from build123d import *

# Parameters (mm, degrees)
EXTRUDE_1_DEPTH = 5


with BuildPart() as part:
    # 草图1 → 凸台-拉伸1 (new body)
    with BuildSketch(Plane(origin=(0, 0, 0), x_dir=(1, 0, 0), z_dir=(0, 1, 0))):
        with BuildLine():
            ThreePointArc((-46.803501746, 8.133377636), (-74.235016913, -2.264931442), (-44.950167705, -4))
            Line((-44.950167705, -4), (-59.407, -4))
            ThreePointArc((-59.407, -4), (-63.361137843, -0.603981718), (-60.601113484, 3.817603042))
            Line((-60.601113484, 3.817603042), (-46.803501746, 8.133377636))
        make_face()
        with BuildLine():
            Line((-60.13775005, 13.480207875), (-65.265019195, 2.816666667))
            ThreePointArc((-65.265019195, 2.816666667), (-65.892913632, 0.427696579), (-65.584160854, -2.023038254))
            Line((-65.584160854, -2.023038254), (-72.827832577, 1.459881143))
            ThreePointArc((-72.827832577, 1.459881143), (-68.690796982, 9.801077165), (-60.13775005, 13.480207875))
        make_face(mode=Mode.SUBTRACT)
        with BuildLine():
            Line((-72.887207875, -0.73075005), (-62.223666667, -5.858019195))
            ThreePointArc((-62.223666667, -5.858019195), (-59.834696579, -6.485913632), (-57.383961746, -6.177160854))
            Line((-57.383961746, -6.177160854), (-60.866881143, -13.420832577))
            ThreePointArc((-60.866881143, -13.420832577), (-69.208077165, -9.283796982), (-72.887207875, -0.73075005))
        make_face(mode=Mode.SUBTRACT)
        with BuildLine():
            Line((-58.67624995, -13.480207875), (-55.320009864, -6.5))
            Line((-55.320009864, -6.5), (-47.574840434, -6.5))
            ThreePointArc((-47.574840434, -6.5), (-52.22107626, -11.428582589), (-58.67624995, -13.480207875))
        make_face(mode=Mode.SUBTRACT)
        with BuildLine():
            ThreePointArc((-57.947118857, 13.420832577), (-53.695607864, 12.232334195), (-50.054812322, 9.735840264))
            Line((-50.054812322, 9.735840264), (-61.347434411, 6.203604944))
            ThreePointArc((-61.347434411, 6.203604944), (-61.388780441, 6.19052068), (-61.430038254, 6.177160854))
            Line((-61.430038254, 6.177160854), (-57.947118857, 13.420832577))
        make_face(mode=Mode.SUBTRACT)
    extrude(amount=EXTRUDE_1_DEPTH)


solid = part.part
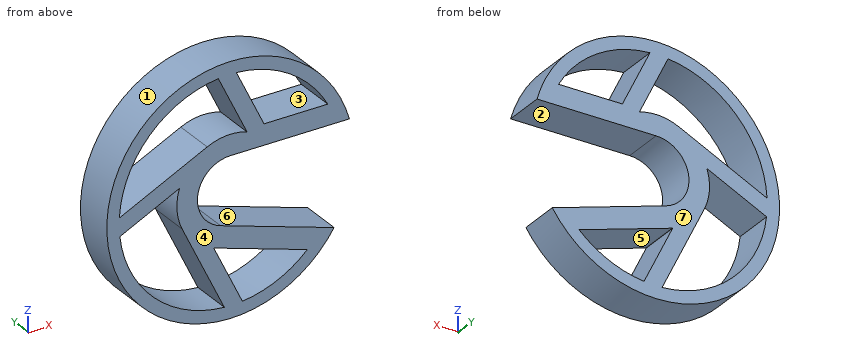
Geometry: final body of the model. Coordinates: model frame, mm. Face numbers are marked on the shaded views. A direction names the side the tool comes from. Coordinates: 2 decimals unless noted, no trailing zeros. Order: outer loops, then holes, each group sorted by start corner. A loop starts at its lowest first (then second) coordinate and runs counter-clockwise, first axis right, second up.
(1) Material intervals for probe 1 along Z at (x, y) = (-71.5, 0.7); probe 2 along X at (y, z) = (2.5, 10.5); probe 3 along Z at (x, y) = (-71, 0.7), sorted ascending.
(2) First-contact query: pin 1 (1.5 mm diameter, centred on x = -49.5, y = 1.5, fed in from -Z); pin 2 (2 mm diameter, centred on x = -68, y = 4, fed in from +Z). Flat tips, straight axial feed; report the tip coordinate or a pass-through.
(3) Section query A-A (x = -54). Return the cut outline in (y, z), plus the area to 3 significant figures.
(4) Section query C-C (z = 0). Return the cut outline in (x, y), plus the area to 3 significant figures.
(5) Section query B-B (y = 3.85). Return the cut outline in (x, z), plus the area to 3 significant figures.
(6) Draft query along Z for the marked faces 1, 2, 3 and 4. Return one class per face: pulls with the +Z half, pulls with the -Z half, needs draft (parallel to the pull), parting line crosses it, or undercut.
(7) Section query D-D (x = -68). Return the cut outline in (y, z), plus the area to 3 significant figures.
(8) Access query for the marked faces 5, 6 and 7. Directions: +Z, -Z, +X, -X, +Y, -Y. A direction counts if a zero-diameter tool reaches every point of the face in a straight line with its end or side. Return the directions, or none.
Solution:
1. probe 1: z = -8.87 to -6, -0.82 to 1.4, 6 to 8.87
1. probe 2: x = -70.12 to -67.89, -59.46 to -57.24, -50.92 to -48.69
1. probe 3: z = -9.52 to -6.92, -0.58 to 1.64, 6.92 to 9.52
2. pin 1: stops at z = -11.88
2. pin 2: stops at z = 12.94
3. outline: (0, -13.99) - (5, -13.99) - (5, -12.37) - (0, -12.37) - close; (0, -8.5) - (5, -8.5) - (5, -5.88) - (0, -5.88) - close; (0, 4) - (5, 4) - (5, 6.5) - (0, 6.5) - close; (0, 12.37) - (5, 12.37) - (5, 13.99) - (0, 13.99) - close
3. area: 41.8 mm2
4. outline: (-74.41, 0) - (-69.79, 0) - (-69.79, 5) - (-74.41, 5) - close; (-65.91, 0) - (-63.41, 0) - (-63.41, 5) - (-65.91, 5) - close
4. area: 35.6 mm2
5. outline: (-60.6, -3.82) arc R4 cw to (-59.41, 4) - (-44.95, 4) arc R15 ccw (long way) to (-46.8, -8.13) - close; hole (-72.89, 0.73) - (-62.22, 5.86) arc R6.5 cw to (-57.38, 6.18) - (-60.87, 13.42) arc R13.5 ccw to start; hole (-72.83, -1.46) arc R13.5 ccw to (-60.14, -13.48) - (-65.27, -2.82) arc R6.5 cw to (-65.58, 2.02) - close; hole (-61.43, -6.18) - (-57.95, -13.42) arc R13.5 ccw to (-50.05, -9.74) - (-61.35, -6.2) arc R6.5 cw to start; hole (-58.68, 13.48) - (-55.32, 6.5) - (-47.57, 6.5) arc R13.5 ccw to start
5. area: 267 mm2
6. face 1: parting line crosses it
6. face 2: undercut
6. face 3: undercut
6. face 4: needs draft
7. outline: (0, -12.29) - (5, -12.29) - (5, -10.41) - (0, -10.41) - close; (0, 0.86) - (5, 0.86) - (5, 3.08) - (0, 3.08) - close; (0, 10.41) - (5, 10.41) - (5, 12.29) - (0, 12.29) - close
7. area: 29.9 mm2
8. face 5: +Y, -Y
8. face 6: +X, +Y, -Y
8. face 7: +Z, -Z, +X, -X, +Y
